from build123d import *

# Parameters (mm, degrees)
SKETCH_W        = 43
SKETCH_H        = 32
PAD_DEPTH       = 30
SKETCH001_W     = 39.5
SKETCH001_H     = 28.4
POCKET_DEPTH    = 28
POCKET001_DEPTH = 32.001
SKETCH003_W     = 35.5
SKETCH003_H     = 24.4
POCKET002_DEPTH = 2.001
POCKET003_DEPTH = 43.001


with BuildPart() as part:
    # Sketch → Pad (new body)
    with BuildSketch(Plane.XY):
        Rectangle(SKETCH_W, SKETCH_H)
    extrude(amount=PAD_DEPTH)

    # Sketch001 → Pocket (cut)
    with BuildSketch(Plane.XY.offset(30)):
        Rectangle(SKETCH001_W, SKETCH001_H)
    extrude(amount=-POCKET_DEPTH, mode=Mode.SUBTRACT)

    # Sketch002 → Pocket001 (cut, through all)
    with BuildSketch(Plane.XZ.offset(16)):
        with BuildLine():
            Line((-11, 30), (11, 30))
            Line((11, 30), (11, 20.499955))
            ThreePointArc((-11, 20.499955), (0, 9.5), (11, 20.499955))
            Line((-11, 20.499955), (-11, 30))
        make_face()
    extrude(amount=-POCKET001_DEPTH, mode=Mode.SUBTRACT)

    # Sketch003 → Pocket002 (cut, through all)
    with BuildSketch(Plane.XY.offset(2)):
        Rectangle(SKETCH003_W, SKETCH003_H)
    extrude(amount=-POCKET002_DEPTH, mode=Mode.SUBTRACT)

    # Sketch004 → Pocket003 (cut, through all)
    with BuildSketch(Plane(origin=(-21.5, 0, 0), x_dir=(0, -1, 0), z_dir=(-1, 0, 0))):
        Polygon((-12.5, 30), (12.5, 30), (9, 12), (-9, 12), align=None)
    extrude(amount=-POCKET003_DEPTH, mode=Mode.SUBTRACT)


solid = part.part
Read the model definition and answer for the solid it produces. Units are mm, in the model's axes. A direction names the side the tool comes from. Give positions to 0.01 mm unless a question says otherwise; leave off trailing zeros. Write each loop counter-clockwise with the first axis right and the second up, starting at its lowest first coordinate (ties: lowest second). Pieces come first, ordered by that corner, then holes. Notation, with made-up numbers: M 26,21.25 L 51,21.25 A15 cw 51,44.25 Z; hole C 45.5,36 d9. An arc over 180 degrees is marked long. One line per item, written item: value. Start each with the question number.
(1) Flat-ended cylindrical pins translate along their axes: pin 1 Ø8 at (y, z) = (10, 24.5) entering from +X; pin 2 Ø0.5 at (x, y) = (-20.5, 4) entering from +Z. Find the tip coordinate at first contact, or state that the pin passes through.
(2) Find section B-B (y = -8.5). Determine the outline of the cut face in (x, z), plus the area to 3 significant figures.
(3) Find the intervals of material crossed by line 1 (X direction, y = 5, z = 10); line 2 (Y direction, x = -0.5, z = 7); line 3 (Z direction, x = 3.5, y = -14), in increasing order.
(4) Find section A-A (x = 16.5). Determine the outline of the cut face in (y, z), plus the area to 3 significant figures.
(5) A tool of negligible diameter and unlimited length cuts with its end or side. For faces 4 (the flat face through (19.75, 0, 10)), 5 (the flat face through (17.75, 0, 1)), 6 (the flat face through (21, 0, 12)), 7 (the flat face through (-11, -15, 25)), from which of +Z, -Z, +X, -X, +Y, -Y can it reach the whole face along a straight path? Write none if from no direction.
(6) Determine the mould class of faces 1 (the cylindrical face through (-0.2, -15.1, 9.5)), 2 (the flat face through (0, -16, 8)), 3 (the flat face through (-20.637, -10.774, 21.126)) for opening direction Y: pulls with the +Y half, pulls with the -Y half, needs draft (parallel to the pull), parting line crosses it, or undercut.
(7) Find section D-D (z = 2.5). Determine the outline of the cut face in (x, y).
(8) Find section C-C (z = 18.75). Determine the outline of the cut face in (x, y).
Results below:
1. pin 1: stops at x = 21.5
1. pin 2: stops at z = 12
2. outline: M -21.5,0 L -17.75,0 L -17.75,2 L -19.75,2 L -19.75,12 L -21.5,12 Z; M 17.75,0 L 21.5,0 L 21.5,12 L 19.75,12 L 19.75,2 L 17.75,2 Z
2. area: 50.0 mm^2
3. line 1: x = -21.5 to -19.75, 19.75 to 21.5
3. line 2: y = -16 to -14.2, 14.2 to 16
3. line 3: z = 0 to 2
4. outline: M -16,0 L -12.2,0 L -12.2,2 L -14.2,2 L -14.2,30 L -16,30 Z; M 12.2,0 L 16,0 L 16,30 L 14.2,30 L 14.2,2 L 12.2,2 Z
4. area: 116 mm^2
5. face 4: +Z
5. face 5: +Z, -Z
5. face 6: +Z, +X, -X
5. face 7: +Z, +Y, -Y
6. face 1: needs draft
6. face 2: pulls with the -Y half
6. face 3: undercut
7. outline: M -21.5,-16 L 21.5,-16 L 21.5,16 L -21.5,16 Z; hole M -19.75,-14.2 L 19.75,-14.2 L 19.75,14.2 L -19.75,14.2 Z
8. outline: M -21.5,-16 L -10.86,-16 L -10.86,-14.2 L -19.75,-14.2 L -19.75,-10.31 L -21.5,-10.31 Z; M -21.5,10.31 L -19.75,10.31 L -19.75,14.2 L -10.86,14.2 L -10.86,16 L -21.5,16 Z; M 10.86,-16 L 21.5,-16 L 21.5,-10.31 L 19.75,-10.31 L 19.75,-14.2 L 10.86,-14.2 Z; M 10.86,14.2 L 19.75,14.2 L 19.75,10.31 L 21.5,10.31 L 21.5,16 L 10.86,16 Z
